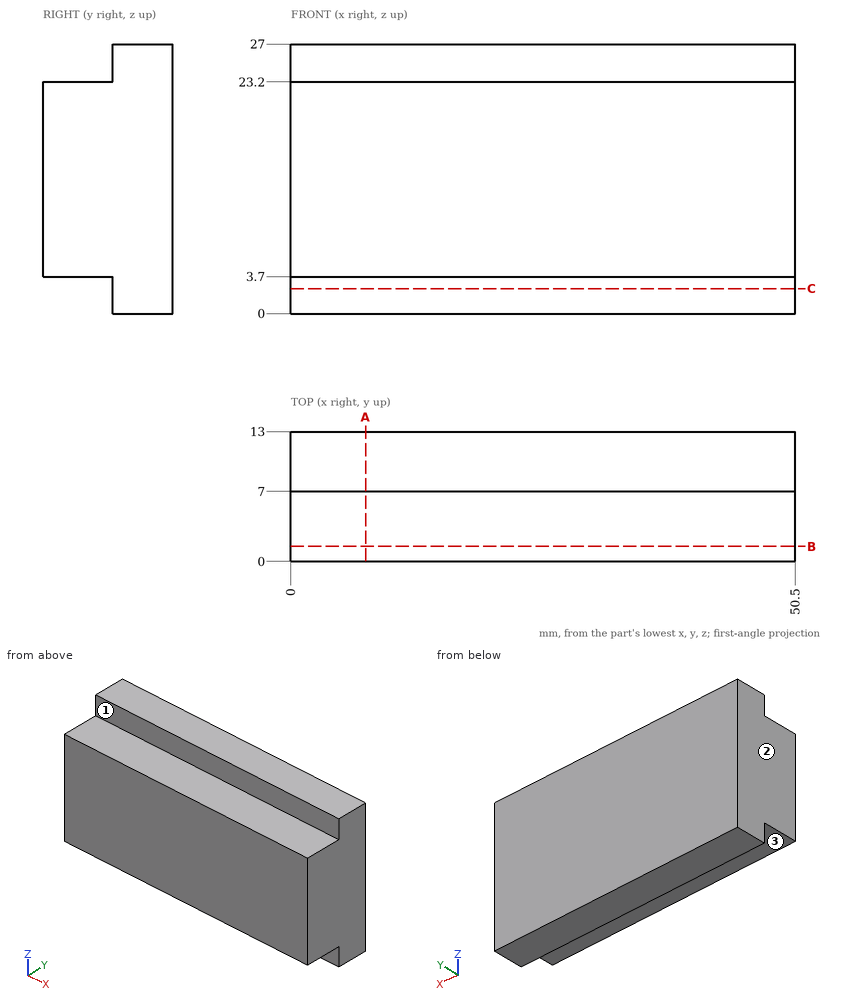
Here's the drawing with two shaded views (mm, measured from the low corner). I have some questions. A direction names the side the tool comes from. Coordinates: 2 decimals unless noted, no trailing zeros. Write each loop counter-clockwise with the first axis right and the second up, starting at its lowest first coordinate (ties: lowest second). Pieces come first, ordered by that corner, then holes. Notation, with made-up numbers: (-13, 30) -> (34, 30) arc R9 cw to (34, 40) -> close; hole circle Ø3 at (3, -36.75). An arc over 180 degrees is marked (long way). Write item = value, one per line. Start each with the question number.
(1) I need wall thicknesses on line 1 (Y direction, x = 30.5, z = 24.5); line 2 (Z direction, x = 17.5, y = 2). Which ranges of each line are inside material? Lowest first, please. Write a range as [from, to].
(2) I want a section at C-C (z = 2.5). Please give me the cut outline in (x, y).
(3) Which directions (+Z, -Z, +X, -X, +Y, -Y) give clear straight access to the entire face, cutting with the end or side of a thin tool? Please do the marked faces 1, 2 and 3.
(4) I want a section at B-B (y = 1.5). Please give me the cut outline in (x, z).
(5) I want a section at A-A (x = 7.5). Please give me the cut outline in (y, z).
(6) Will these pins go through, and if not, where does the flat tip stop? pin 1 (3.5 mm diameter, centred on x = 16, y = 2, fed in from +Z); pin 2 (3 mm diameter, centred on x = 23.5, z = 1, fed in from -Y); pin 3 (7.5 mm diameter, centred on x = 22.5, y = 2, fed in from -Z).
Result set:
q1.line_1 = [7, 13]
q1.line_2 = [3.7, 23.2]
q2.outline = (0, 7) -> (50.5, 7) -> (50.5, 13) -> (0, 13) -> close
q3.face_1 = +Z, +X, -X, -Y
q3.face_2 = +Z, -Z, -X, +Y, -Y
q3.face_3 = -Z, +X, -X, -Y
q4.outline = (0, 3.7) -> (50.5, 3.7) -> (50.5, 23.2) -> (0, 23.2) -> close
q5.outline = (0, 3.7) -> (7, 3.7) -> (7, 0) -> (13, 0) -> (13, 27) -> (7, 27) -> (7, 23.2) -> (0, 23.2) -> close
q6.pin_1 = 23.2
q6.pin_2 = 7
q6.pin_3 = 3.7
